```python
from build123d import *

# Parameters (mm, degrees)
SKETCH001_W          = 4.2
SKETCH001_H          = 5.6
POCKET_DEPTH         = 2.5
SKETCH002_R          = 0.7874
POCKET001_DEPTH      = 14.501
SKETCH004_W          = 0.5
SKETCH004_H          = 11.942059
SKETCH004_H_2        = 6.122161
POCKET003_DEPTH      = 5
POCKET003_DEPTH_BACK = -5


with BuildPart() as part:
    # Sketch → Revolution (revolve)
    with BuildSketch(Plane.XZ):
        Polygon((2.5, 0), (4, 0), (4, -4), (0, -4), (0, 0), (0, 10.5), (1.9, 10.5), (1.4, 9.15), (2.6, 3.5), (2.5, 2.5), align=None)
    revolve(axis=Axis((0, 0, 0), (0, 0, 1)))

    # Sketch001 (on Face5 of Revolution) → Pocket (cut)
    with BuildSketch(Plane(origin=(0, 0, -4), x_dir=(1, 0, 0), z_dir=(0, 0, -1))):
        Rectangle(SKETCH001_W, SKETCH001_H)
    extrude(amount=-POCKET_DEPTH, mode=Mode.SUBTRACT)

    # Sketch002 (on Face6 of Pocket) → Pocket001 (cut, through all)
    with BuildSketch(Plane(origin=(0, 0, 10.5), x_dir=(-1, 0, 0), z_dir=(0, 0, 1))):
        Circle(SKETCH002_R)
    extrude(amount=-POCKET001_DEPTH, mode=Mode.SUBTRACT)

    # Sketch004 → Pocket003 (cut, two sides)
    with BuildSketch(Plane.XZ) as pocket003_sk:
        with Locations((0, 6.971029)):
            Rectangle(SKETCH004_W, SKETCH004_H)
        with Locations((0, -13.475635)):
            Rectangle(SKETCH004_W, SKETCH004_H_2)
    extrude(amount=-POCKET003_DEPTH, mode=Mode.SUBTRACT)
    extrude(pocket003_sk.sketch, amount=-POCKET003_DEPTH_BACK, mode=Mode.SUBTRACT)


solid = part.part
```
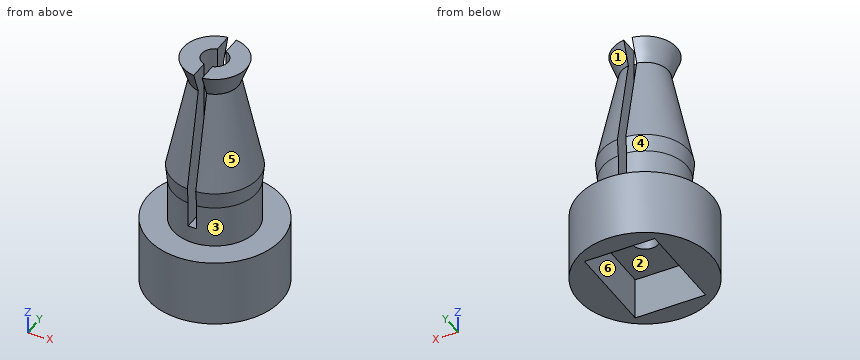
Part model, mm, in its own coordinate system. Face numbers are marked on the shaded views. A direction names the side the tool comes from. Round coordinates to 2 decimals unless told otherwise and drop trailing zeros. Loops run counter-clockwise (first coordinate to the right, second up) from the corner with the lowest first, then second, coordinate; pieces in that order, holes last.
1. Slice it at D-D (z = 9.5). Give the cut face in (x, y), and give its area (3 significant figures).
Solutions:
outline: (-0.25, -1.51) - (-0.25, -0.75) arc R0.79 cw to (-0.25, 0.75) - (-0.25, 1.51) arc R1.53 ccw to start; (0.25, -1.51) arc R1.53 ccw to (0.25, 1.51) - (0.25, 0.75) arc R0.79 cw to (0.25, -0.75) - close
area: 4.65 mm2
2. 3-axis set-ups, long thin cutter, end or side, ignore diameter. For the marked faces 4, 5 and 6: which of +Z, -Z, +X, -X, +Y, -Y reach the whole face in a straight line?
Solutions:
face 4: -X
face 5: +X
face 6: -Z
3. Flat gauge pins, fed straight in: pin 1 (2 mm diameter, centred on y = -1.5, z = -3.5, fed in from +X); pin 2 (0.9 mm diameter, centred on y = 1.5, z = 5, fed in from -X); pin 3 (1.5 mm diameter, centred on y = 2, z = 8, fed in from +X); pin 4 (3.5 mm diameter, centred on x = -1, y = -1, fed in from -Z). Where does each tip first touch, or does it go through?
Solutions:
pin 1: stops at x = 3.97
pin 2: stops at x = -2.05
pin 3: stops at x = 1.1
pin 4: stops at z = -4
4. Slice it at B-B (y = 0). Give the cut face in (x, z).
Solutions:
outline: (-4, -4) - (-2.1, -4) - (-2.1, -1.5) - (-0.79, -1.5) - (-0.79, 10.5) - (-1.9, 10.5) - (-1.4, 9.15) - (-2.6, 3.5) - (-2.5, 2.5) - (-2.5, 0) - (-4, 0) - close; (0.79, -1.5) - (2.1, -1.5) - (2.1, -4) - (4, -4) - (4, 0) - (2.5, 0) - (2.5, 2.5) - (2.6, 3.5) - (1.4, 9.15) - (1.9, 10.5) - (0.79, 10.5) - close
5. Slice it at A-A (x = 0). Give the cut face in (y, z), and give its area (3 significant figures).
Solutions:
outline: (-4, -4) - (-2.8, -4) - (-2.8, -1.5) - (-0.79, -1.5) - (-0.79, 1) - (-2.5, 1) - (-2.5, 0) - (-4, 0) - close; (0.79, -1.5) - (2.8, -1.5) - (2.8, -4) - (4, -4) - (4, 0) - (2.5, 0) - (2.5, 1) - (0.79, 1) - close
area: 19.1 mm2
6. Slice it at C-C (z = -2.75). Give the cut face in (x, y), and give its area (3 significant figures).
Solutions:
outline: circle Ø8 at (0, 0); hole (-2.1, -2.8) - (2.1, -2.8) - (2.1, 2.8) - (-2.1, 2.8) - close
area: 26.7 mm2
7. Two-plate mould, pull along X, no slides. Class the marked faces 1, 2 and 3: pulls with the +X half, pulls with the -X half, needs draft (parallel to the pull), parting line crosses it, or undercut.
Solutions:
face 1: pulls with the +X half
face 2: undercut
face 3: parting line crosses it
8. Drill centre lines: line 1 along X through (y, z) = (0, 1); line 2 along Z through (x, y) = (-1.25, -3.25); line 3 along Y through (x, z) = (1.5, -2.5). Where is each one in solid material? Low to high.
Solutions:
line 1: x = -2.5 to -0.79, 0.79 to 2.5
line 2: z = -4 to 0
line 3: y = -3.71 to -2.8, 2.8 to 3.71
